The listing builds one solid part. Answer for the finished solid, in the listing's coordinates (mm). Give positions to 0.01 mm unless a question says otherwise; leave off trailing zeros. Write each loop counter-clockwise with the first axis right and the second up, starting at its lowest first coordinate (ties: lowest second). Pieces come first, ordered by that corner, then holes. Notation, with made-up numbers: (17, -12.5) -> (63, -12.5) arc R20 ccw to (63, 9.5) -> close; hole circle Ø9 at (40, 89.25). An arc over 180 degrees is marked (long way). One line per question, with ' | ' between items.
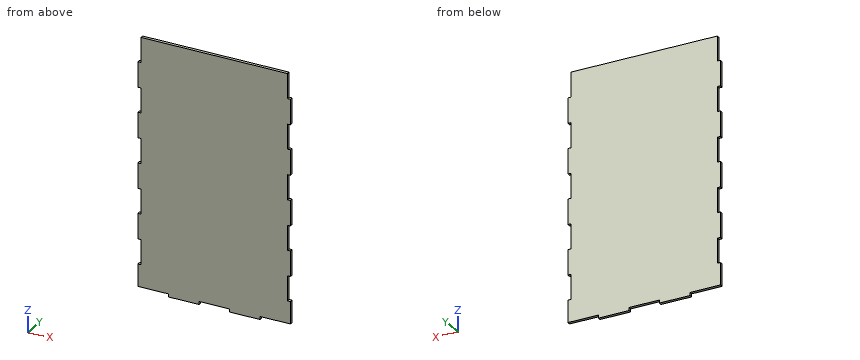
from build123d import *

# Parameters (mm, degrees)
BOSS_EXTRUDE1_DEPTH = 3


with BuildPart() as part:
    # Sketch1 → Boss-Extrude1 (new body)
    with BuildSketch(Plane(origin=(0, 0, 0), x_dir=(1, 0, 0), z_dir=(0, 1, 0))):
        Polygon((3, 24.8), (3, 0), (147, 0), (147, 24.8), (150, 24.8), (150, 50), (147, 50), (147, 74.8), (150, 74.8), (150, 100), (147, 100), (147, 124.8), (150, 124.8), (150, 150), (147, 150), (147, 174.8), (150, 174.8), (150, 200), (147, 200), (147, 224.8), (150, 224.8), (150, 247), (120.2, 247), (120.2, 250), (89.9, 250), (89.9, 247), (60.1, 247), (60.1, 250), (29.8, 250), (29.8, 247), (0, 247), (0, 224.8), (3, 224.8), (3, 200), (0, 200), (0, 174.8), (3, 174.8), (3, 150), (0, 150), (0, 124.8), (3, 124.8), (3, 100), (0, 100), (0, 74.8), (3, 74.8), (3, 50), (0, 50), (0, 24.8), align=None)
    extrude(amount=BOSS_EXTRUDE1_DEPTH)


solid = part.part
Item 1: Find section A-A (z = -114). Write down the section's boundary in (x, y), then the cut area to 3 significant figures.
Answers below:
outline: (3, 0) -> (147, 0) -> (147, 3) -> (3, 3) -> close | area: 432 mm²
Item 2: Consider line 1 (Z direction, x = 144.5, y = 2.3); line 2 (X direction, y = 0.2, z = -124). Determine where each line is inside the solid, lowest interval first. Write a range as [from, to].
Answers below:
line 1: [-247, 0] | line 2: [3, 147]
Item 3: Flat-ended cylindrical pins translate along their axes: pin 1 (0.9 mm diameter, centred on x = 1.5, y = 2, fed in from -Z); pin 2 (10 mm diameter, centred on x = 113.5, z = -154.5, fed in from -Y); pin 3 (1.5 mm diameter, centred on x = 149, y = 1, fed in from +Z); pin 4 (0.9 mm diameter, centred on y = 2, z = -66, fed in from +X). Find the tip coordinate at first contact, or state that the pin passes through.
Answers below:
pin 1: z = -247 | pin 2: y = 0 | pin 3: z = -24.8 | pin 4: x = 147
